```python
from build123d import *

# Parameters (mm, degrees)
SKETCH1_W           = 2
SKETCH1_H           = 2
SKETCH1_W_2         = 7
SKETCH1_H_2         = 5
BOSS_EXTRUDE2_DEPTH = 2
FILLET1_R           = 10
FILLET2_R           = 10
FILLET3_R           = 5
FILLET4_R           = 5


with BuildPart() as part:
    # Sketch1 → Boss-Extrude2 (new body)
    with BuildSketch(Plane.XY):
        with BuildLine():
            Line((-42.5, 0), (-35.5, 0))
            Line((-35.5, 0), (-35.5, 2))
            ThreePointArc((-35.5, 2), (-37.621320344, 7.121320344), (-32.5, 5))
            Line((-32.5, 5), (-30.5, 5))
            Line((-30.5, 5), (-30.5, 12))
            Line((-30.5, 12), (-42.5, 12))
            Line((-42.5, 12), (-42.5, 0))
        make_face()
        with Locations((-40.5, 10)):
            Rectangle(SKETCH1_W, SKETCH1_H, mode=Mode.SUBTRACT)
        Polygon((-18.5, -5), (-35.5, -5), (-42.5, -5), (-42.5, -9), (-22.5, -9), (-22.5, -10), (-18.5, -10), (-18.5, -9), align=None)
        with Locations((-20.5, -8)):
            Rectangle(SKETCH1_W, SKETCH1_H, mode=Mode.SUBTRACT)
        with Locations((-39, -2.5)):
            Rectangle(SKETCH1_W_2, SKETCH1_H_2)
        with BuildLine():
            Line((-35.5, 0), (-35.5, -5))
            Line((-35.5, -5), (-18.5, -5))
            Line((-18.5, -5), (-5, -5))
            Line((-5, -5), (-5, 0))
            Line((-5, 0), (-10, 0))
            Line((-10, 0), (-13, 0))
            Line((-13, 0), (-13, 5))
            Line((-13, 5), (-30.5, 5))
            Line((-30.5, 5), (-32.5, 5))
            ThreePointArc((-32.5, 5), (-33.378679656, 2.878679656), (-35.5, 2))
            Line((-35.5, 2), (-35.5, 0))
        make_face()
        Polygon((-10, 0), (-5, 0), (5, 0), (10, 0), (10, 5), (-10, 5), align=None)
        Polygon((35.5, -5), (18.5, -5), (18.5, -9), (18.5, -10), (22.5, -10), (22.5, -9), (42.5, -9), (42.5, -5), align=None)
        with Locations((20.5, -8)):
            Rectangle(SKETCH1_W, SKETCH1_H, mode=Mode.SUBTRACT)
        with Locations((39, -2.5)):
            Rectangle(SKETCH1_W_2, SKETCH1_H_2)
        with BuildLine():
            Line((35.5, 2), (35.5, 0))
            Line((35.5, 0), (42.5, 0))
            Line((42.5, 0), (42.5, 12))
            Line((42.5, 12), (30.5, 12))
            Line((30.5, 12), (30.5, 5))
            Line((30.5, 5), (32.5, 5))
            ThreePointArc((32.5, 5), (35.5, 8), (38.5, 5))
            ThreePointArc((38.5, 5), (37.621320344, 2.878679656), (35.5, 2))
        make_face()
        with Locations((40.5, 10)):
            Rectangle(SKETCH1_W, SKETCH1_H, mode=Mode.SUBTRACT)
        with BuildLine():
            Line((5, 0), (5, -5))
            Line((5, -5), (18.5, -5))
            Line((18.5, -5), (35.5, -5))
            Line((35.5, -5), (35.5, 0))
            Line((35.5, 0), (35.5, 2))
            ThreePointArc((35.5, 2), (33.378679656, 2.878679656), (32.5, 5))
            Line((32.5, 5), (30.5, 5))
            Line((30.5, 5), (13, 5))
            Line((13, 5), (13, 0))
            Line((13, 0), (10, 0))
            Line((10, 0), (5, 0))
        make_face()
    extrude(amount=BOSS_EXTRUDE2_DEPTH)

    # Fillet1
    fillet1_edges = [part.edges().sort_by_distance(p)[0] for p in [
        (-42.5, -9, 1),
    ]]
    fillet(fillet1_edges, radius=FILLET1_R)

    # Fillet2
    fillet2_edges = [part.edges().sort_by_distance(p)[0] for p in [
        (42.5, -9, 1),
    ]]
    fillet(fillet2_edges, radius=FILLET2_R)

    # Fillet3
    fillet3_edges = [part.edges().sort_by_distance(p)[0] for p in [
        (-30.5, 12, 1),
    ]]
    fillet(fillet3_edges, radius=FILLET3_R)

    # Fillet4
    fillet4_edges = [part.edges().sort_by_distance(p)[0] for p in [
        (30.5, 12, 1),
    ]]
    fillet(fillet4_edges, radius=FILLET4_R)


solid = part.part
```
Part model, mm, in its own coordinate system. A direction names the side the tool comes from. Give positions to 0.01 mm unless a question says otherwise; leave off trailing zeros. Order: outer loops, then holes, each group sorted by start corner. A loop starts at its lowest first (then second) coordinate and runs counter-clockwise, first axis right, second up. Notation, with made-up numbers: (6.5, 81.5) - (37.5, 81.5) arc R30 ccw to (37.5, 110.5) - close; hole circle Ø6 at (-35, 88.5). An arc over 180 degrees is marked (long way). Use one line per item in the form item = value.
Item 1: Slice it at C-C on z = 1.35. Count the separate pieces of the cut face and the enclosed holes in it, and give its area (3 significant figures).
Solution:
separate_pieces = 1
enclosed_holes = 6
area = 1,010 mm2
Item 2: Two-plate mould, pull along Y, no slides. Class faces 4 (the face through (-21, -9, 1)), 5 (the face through (22, 5, 1)), 6 (the face through (-39.65, -5.99, 1.01)), 7 (the face through (41.5, 10, 1)): released by +Y, released by -Y, zero draft, split by the parting line, or undercut.
Solution:
face_4 = undercut
face_5 = released by +Y
face_6 = released by -Y
face_7 = undercut
Item 3: Which spindle directions (+Z, -Z, +X, -X, +Y, -Y) get a long thin tool onto all of the face, cutting with end or side? Do faces 1 (the face through (18.5, -7, 1)), 2 (the face through (31.93, 10.5, 1.01)), 3 (the face through (-39.5, 10, 1)). Say none if no direction does.
Solution:
face_1 = +Z, -Z, -Y
face_2 = +Z, -Z, +Y
face_3 = +Z, -Z
Item 4: Probe probe 1 along X at (y, z) = (1, 0.2); probe 2 along X at (y, z) = (4.75, 1.55); probe 3 along Y at (x, z) = (-21, 0.7). List the from-to ranges inside material, lowest first. Write a range as from..to.
Solution:
probe_1 = -42.5..-13, -10..10, 13..42.5
probe_2 = -42.5..-38.49, -32.51..-13, -10..10, 13..32.51, 38.49..42.5
probe_3 = -10..-9, -7..5
Item 5: Slice it at D-D on y = 2.75. Give the cut face in (x, z), and give its area (3 significant figures).
Solution:
outline = (-42.5, 0) - (-37.48, 0) - (-37.48, 2) - (-42.5, 2) - close; (-33.52, 0) - (-13, 0) - (-13, 2) - (-33.52, 2) - close; (-10, 0) - (10, 0) - (10, 2) - (-10, 2) - close; (13, 0) - (33.52, 0) - (33.52, 2) - (13, 2) - close; (37.48, 0) - (42.5, 0) - (42.5, 2) - (37.48, 2) - close
area = 142 mm2
Item 6: Pin check, flat tip, straight feed: pin 1 Ø1 at (x, z) = (-20.5, 1) entering from +Y. Stop position of the tip, or through.
Solution:
pin_1 = 5
Item 7: Slice it at A-A on y = -2.5. Give the cut face in (x, z), and give its area (3 significant figures).
Solution:
outline = (-41.87, 0) - (-5, 0) - (-5, 2) - (-41.87, 2) - close; (5, 0) - (41.87, 0) - (41.87, 2) - (5, 2) - close
area = 147 mm2
Item 8: Slice it at B-B on y = -8.25. Give the cut face in (x, z).
Solution:
outline = (-36.3, 0) - (-21.5, 0) - (-21.5, 2) - (-36.3, 2) - close; (-19.5, 0) - (-18.5, 0) - (-18.5, 2) - (-19.5, 2) - close; (18.5, 0) - (19.5, 0) - (19.5, 2) - (18.5, 2) - close; (21.5, 0) - (36.3, 0) - (36.3, 2) - (21.5, 2) - close
